CAD build for the part. Positions are in the model's coordinates, mm. A direction names the side the tool comes from. Round coordinates to 2 decimals unless told otherwise and drop trailing zeros. Loops run counter-clockwise (first coordinate to the right, second up) from the corner with the lowest first, then second, coordinate; pieces in that order, holes last. Notation, with made-up numbers: M -26,-3.5 L 12,-3.5 A11 cw 12,10.5 Z; hole C 81.25,44 d2. An arc over 180 degrees is marked long. Use a Markdown table: item, result. Add a question column.
(1) Wall check: L1, parallel to Y at x = -41.5, z = 12.5; L2, parallel to X at y = 8, z = 39.5; L3, parallel to Z at x = -50.5, y = 30. Give the ranges that are in metal, low to high.
(2) Band-saw the part on A-A, the plane x = 59.5. Write the cut outline in (y, z), and give its area (3 significant figures).
(3) Band-saw the part on B-B, the plane y = 39.5. Write the cut outline in (x, z), and give its area (3 significant figures).
(4) Flat gauge pins, fed straight in: P1, Ø3, axis at y = -27, z = 47.5, coming from the -X side; P2, Ø5, axis at x = 41, z = 43.5, coming from the -Y side; P3, Ø1.5, axis at y = 42.5, z = 56.5, coming from the -X side. Where does each tip first touch, or does it go through?
(5) Band-saw the part on D-D, the plane x = -7.5. Write the cut outline in (y, z), and give its area (3 significant figures).
(6) Two-plate mould, pull along X, no slides. Class faces 5 (the face through (-37, -58.054, 15)), 6 (the face through (78.561, -1, 15)), 7 (the face through (38.211, -39, 5)): released by +X, released by -X, zero draft, split by the parting line, or undercut.
(7) Band-saw the part on C-C, the plane y = 6. Write the cut outline in (x, z), and give its area (3 significant figures).
(8) Which spindle directions (+Z, -Z, +X, -X, +Y, -Y) get a long thin tool onto all of the face, cutting with end or side? Do faces 1 (the face through (8, 56.946, 15)), 2 (the face through (28.561, -26, 35)), 3 (the face through (48, -28.845, 19)), 4 (the face through (62, 16.946, 15)). Say none if no direction does.
from build123d import *

# Parameters (mm, degrees)
SKETCH_1_W          = 140
SKETCH_1_H          = 115
SKETCH_1_R          = 36
SKETCH_1_W_2        = 20
SKETCH_1_H_2        = 20
EXTRUDE_1_DEPTH     = 30
SKETCH_2_R          = 40
CUT_EXTRUDE_1_DEPTH = 10
SKETCH_10_R         = 41
SKETCH_10_R_2       = 36
EXTRUDE_3_DEPTH     = 40
CUT_EXTRUDE_2_REACH = 117
SKETCH_3_W          = 40
SKETCH_3_H          = 80
SKETCH_4_R          = 3.75
SKETCH_4_W          = 18.75
SKETCH_4_H          = 7.5
CUT_EXTRUDE_3_DEPTH = 15
SKETCH_6_W          = 9.65
SKETCH_6_H          = 20.5
CUT_EXTRUDE_4_DEPTH = 31
SKETCH_7_W          = 29
SKETCH_7_H          = 20.5
CUT_EXTRUDE_5_DEPTH = 21
SKETCH_11_W         = 7
SKETCH_11_H         = 8
CUT_EXTRUDE_6_DEPTH = 10


with BuildPart() as part:
    # 草圖1 → 填料-伸長1 (new body)
    with BuildSketch(Plane.XY):
        with Locations((8.56146046, -0.554151625)):
            Rectangle(SKETCH_1_W, SKETCH_1_H)
        with Locations((8.56146046, 6.945848375)):
            Circle(SKETCH_1_R, mode=Mode.SUBTRACT)
        with Locations((-45.43853954, 6.945848375)):
            Rectangle(SKETCH_1_W_2, SKETCH_1_H_2, mode=Mode.SUBTRACT)
        with Locations((62.56146046, 6.945848375)):
            Rectangle(SKETCH_1_W_2, SKETCH_1_H_2, mode=Mode.SUBTRACT)
    extrude(amount=EXTRUDE_1_DEPTH)

    # 草圖2 → 除料-伸長1 (cut)
    with BuildSketch(Plane(origin=(0, 0, 0), x_dir=(-1, 0, 0), z_dir=(0, 0, -1))):
        with Locations((-8.56146046, 6.945848375)):
            Circle(SKETCH_2_R)
    extrude(amount=-CUT_EXTRUDE_1_DEPTH, mode=Mode.SUBTRACT)

    # 草圖10 → 填料-伸長3 (add)
    with BuildSketch(Plane.XY.offset(30)):
        with Locations((8.56146046, 6.945848375)):
            Circle(SKETCH_10_R)
        with Locations((8.56146046, 6.945848375)):
            Circle(SKETCH_10_R_2, mode=Mode.SUBTRACT)
    extrude(amount=EXTRUDE_3_DEPTH)

    # 草圖3 → 除料-伸長2 (cut, up to next)
    with BuildSketch(Plane.XZ.offset(58.054151625), mode=Mode.PRIVATE) as cut_extrude_2_sk1:
        with Locations((8.56146046, 40)):
            Rectangle(SKETCH_3_W, SKETCH_3_H)
    cut_extrude_2_tool1 = extrude(cut_extrude_2_sk1.sketch, amount=-CUT_EXTRUDE_2_REACH, mode=Mode.PRIVATE) & part.part
    add(cut_extrude_2_tool1.solids().sort_by_distance((8.56146, -58.054152, 40))[0], mode=Mode.SUBTRACT)

    # 草圖4 → 除料-伸長3 (cut)
    with BuildSketch(Plane(origin=(-11.43853954, 0, 0), x_dir=(0, 0, -1), z_dir=(1, 0, 0))):
        with Locations((-11.25, -39.095211961)):
            Circle(SKETCH_4_R)
        with Locations((-20.625, -39.095211961)):
            Rectangle(SKETCH_4_W, SKETCH_4_H)
    extrude(amount=-CUT_EXTRUDE_3_DEPTH, mode=Mode.SUBTRACT)

    # 草圖6 → 除料-伸長4 (cut, through all)
    with BuildSketch(Plane.XY.offset(30)):
        with Locations((33.38646046, -39.095211961)):
            Rectangle(SKETCH_6_W, SKETCH_6_H)
    extrude(amount=-CUT_EXTRUDE_4_DEPTH, mode=Mode.SUBTRACT)

    # 草圖7 → 除料-伸長5 (cut)
    with BuildSketch(Plane.XY.offset(30)):
        with Locations((52.71146046, -39.095211961)):
            Rectangle(SKETCH_7_W, SKETCH_7_H)
    extrude(amount=-CUT_EXTRUDE_5_DEPTH, mode=Mode.SUBTRACT)

    # 草圖11 → 除料-伸長6 (cut)
    with BuildSketch(Plane.XY.offset(9)):
        with Locations((60.71146046, -39.095211961)):
            Rectangle(SKETCH_11_W, SKETCH_11_H)
    extrude(amount=-CUT_EXTRUDE_6_DEPTH, mode=Mode.SUBTRACT)


solid = part.part
Return value:
| question | item | result |
|---|---|---|
| 1 | L1 | -58.05 to -3.05, 16.95 to 56.95 |
| 1 | L2 | -32.42 to -27.42, 44.55 to 49.55 |
| 1 | L3 | 0 to 30 |
| 2 | outline | M -58.05,0 L -43.1,0 L -43.1,9 L -49.35,9 L -49.35,30 L -58.05,30 Z; M -35.1,0 L -3.05,0 L -3.05,30 L -28.85,30 L -28.85,9 L -35.1,9 Z; M 16.95,0 L 56.95,0 L 56.95,30 L 16.95,30 Z |
| 2 | area | 2,350 mm^2 |
| 3 | outline | M -61.44,0 L -14.68,0 L -14.68,10 L -6.81,10 L -6.81,70 L -16.36,70 L -16.36,30 L -61.44,30 Z; M 23.93,10 L 31.8,10 L 31.8,0 L 78.56,0 L 78.56,30 L 33.49,30 L 33.49,70 L 23.93,70 Z |
| 3 | area | 3,880 mm^2 |
| 4 | P1 | x = -16.5 |
| 4 | P2 | y = -21.07 |
| 4 | P3 | x = -13.11 |
| 5 | outline | M 39.16,10 L 43.58,10 L 43.58,0 L 56.95,0 L 56.95,30 L 44.67,30 L 44.67,70 L 39.16,70 Z |
| 5 | area | 709 mm^2 |
| 6 | face 5 | zero draft |
| 6 | face 6 | released by +X |
| 6 | face 7 | undercut |
| 7 | outline | M -61.44,0 L -55.44,0 L -55.44,30 L -61.44,30 Z; M -35.44,0 L -31.43,0 L -31.43,10 L -27.43,10 L -27.43,70 L -32.43,70 L -32.43,30 L -35.44,30 Z; M 44.55,10 L 48.55,10 L 48.55,0 L 52.56,0 L 52.56,30 L 49.55,30 L 49.55,70 L 44.55,70 Z; M 72.56,0 L 78.56,0 L 78.56,30 L 72.56,30 Z |
| 7 | area | 1,160 mm^2 |
| 8 | face 1 | +Z, -Z, +X, -X, +Y |
| 8 | face 2 | +Z, -Z, -Y |
| 8 | face 3 | +Z |
| 8 | face 4 | +Z, -Z |
